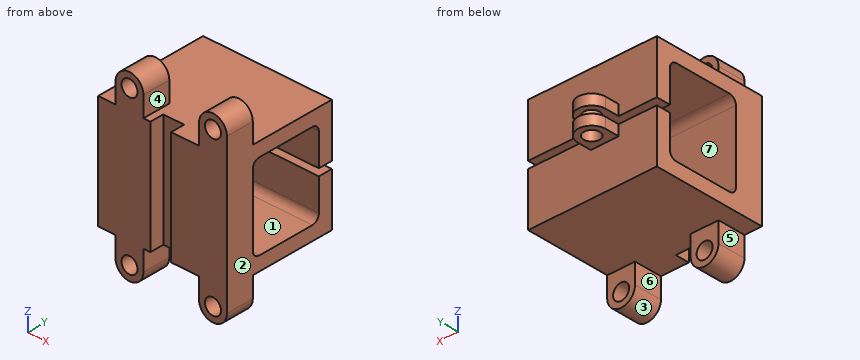
```python
from build123d import *

# Parameters (mm, degrees)
SKETCH_1_W           = 8
SKETCH_1_H           = 5
SKETCH_1_R           = 1.15
EXTRUDE_1_DEPTH      = 4
SKETCH_2_W           = 10.5
SKETCH_2_H           = 8
SKETCH_2_R           = 1.15
EXTRUDE_2_DEPTH      = 7
EXTRUDE_4_DEPTH      = 15
SKETCH_6_R           = 1.15
EXTRUDE_5_DEPTH      = 1.5
EXTRUDE_START        = 2.5
SKETCH_6_2_R         = 1.15
EXTRUDE_6_DEPTH      = 1.5
CUT_EXTRUDE_2_DEPTH  = 3
FILLET_2_R           = 1
SKETCH_9_OUTSIDE_W   = 25.014
SKETCH_9_OUTSIDE_H   = 34.214
SKETCH_9_OUTSIDE_W_2 = 15
SKETCH_9_OUTSIDE_H_2 = 16.2
CUT_EXTRUDE_3_DEPTH  = 36.814522194
SKETCH_12_W          = 16.2
SKETCH_12_H          = 8
CUT_EXTRUDE_5_DEPTH  = 31.608495553
SKETCH_10_W          = 3
SKETCH_10_H          = 2
CUT_EXTRUDE_4_DEPTH  = 31.608495553
SKETCH_11_R          = 1.15
EXTRUDE_7_DEPTH      = 4
EXTRUDE_15_DEPTH     = 3.5


with BuildPart() as part:
    # 草图1 → 凸台-拉伸1 (new body)
    with BuildSketch(Plane(origin=(0, 0, 0), x_dir=(0, 0, -1), z_dir=(1, 0, 0))):
        with Locations((4, 2.5)):
            Rectangle(SKETCH_1_W, SKETCH_1_H)
        with Locations((2, 2.5)):
            Circle(SKETCH_1_R, mode=Mode.SUBTRACT)
        with Locations((6, 2.5)):
            Circle(SKETCH_1_R, mode=Mode.SUBTRACT)
    extrude(amount=EXTRUDE_1_DEPTH)

    # 草图2 → 凸台-拉伸2 (add)
    with BuildSketch(Plane.XZ):
        with Locations((5.25, -4)):
            Rectangle(SKETCH_2_W, SKETCH_2_H)
        with Locations(Location((8, -6, 0), (0, 0, 270))):
            Circle(SKETCH_2_R, mode=Mode.SUBTRACT)
        with Locations(Location((8, -2, 0), (0, 0, 270))):
            Circle(SKETCH_2_R, mode=Mode.SUBTRACT)
    extrude(amount=EXTRUDE_2_DEPTH)

    # 草图5 → 凸台-拉伸4 (add)
    with BuildSketch(Plane.ZY):
        Polygon((14.2, 5), (2, 5), (2, 15.2), (7.6, 15.2), (7.6, 17.2), (0, 17.2), (0, -7), (16.2, -7), (16.2, 17.2), (8.6, 17.2), (8.6, 15.2), (14.2, 15.2), align=None)
    extrude(amount=-EXTRUDE_4_DEPTH)

    # 草图6 → 凸台-拉伸5 (add)
    with BuildSketch(Plane.XY.offset(7.6)):
        with BuildLine():
            Line((2, 19.2), (2, 17.2))
            Line((2, 17.2), (6, 17.2))
            Line((6, 17.2), (6, 19.2))
            ThreePointArc((6, 19.2), (4, 21.2), (2, 19.2))
        make_face()
        with Locations((4, 19.2)):
            Circle(SKETCH_6_R, mode=Mode.SUBTRACT)
    extrude(amount=-EXTRUDE_5_DEPTH)

    # 草图6<2> → 凸台-拉伸6 (add)
    with BuildSketch(Plane.XY.offset(7.6).offset(EXTRUDE_START)):
        with BuildLine():
            Line((2, 19.2), (2, 17.2))
            Line((2, 17.2), (6, 17.2))
            Line((6, 17.2), (6, 19.2))
            ThreePointArc((6, 19.2), (4, 21.2), (2, 19.2))
        make_face()
        with Locations((4, 19.2)):
            Circle(SKETCH_6_2_R, mode=Mode.SUBTRACT)
    extrude(amount=-EXTRUDE_6_DEPTH)

    # 草图8 → 切除-拉伸2 (cut)
    with BuildSketch(Plane(origin=(0, 0, -8), x_dir=(-1, 0, 0), z_dir=(0, 0, -1))):
        Polygon((0, -3), (0, -7), (-4, -7), align=None)
    extrude(amount=-CUT_EXTRUDE_2_DEPTH, mode=Mode.SUBTRACT)

    # 圆角2
    fillet_2_edges = [part.edges().sort_by_distance(p)[0] for p in [
        (7.5, 15.2, 2),
        (7.5, 5, 2),
        (7.5, 5, 14.2),
        (7.5, 15.2, 14.2),
    ]]
    fillet(fillet_2_edges, radius=FILLET_2_R)

    # 草图9 outside → 切除-拉伸3 (cut, through all)
    with BuildSketch(Plane.XZ.offset(7)):
        with Locations((7.5, 4.1)):
            Rectangle(SKETCH_9_OUTSIDE_W, SKETCH_9_OUTSIDE_H)
        with Locations((7.5, 8.1)):
            Rectangle(SKETCH_9_OUTSIDE_W_2, SKETCH_9_OUTSIDE_H_2, mode=Mode.SUBTRACT)
    extrude(amount=-CUT_EXTRUDE_3_DEPTH, mode=Mode.SUBTRACT)

    # 草图12 → 切除-拉伸5 (cut, through all)
    with BuildSketch(Plane(origin=(15, 0, 0), x_dir=(0, 0, -1), z_dir=(1, 0, 0))):
        with Locations((-8.1, -3)):
            Rectangle(SKETCH_12_W, SKETCH_12_H)
    extrude(amount=-CUT_EXTRUDE_5_DEPTH, mode=Mode.SUBTRACT)

    # 草图10 → 切除-拉伸4 (cut, through all)
    with BuildSketch(Plane(origin=(0, 0, 0), x_dir=(-1, 0, 0), z_dir=(0, 0, -1))):
        with Locations((-5.5, 2)):
            Rectangle(SKETCH_10_W, SKETCH_10_H)
    extrude(amount=-CUT_EXTRUDE_4_DEPTH, mode=Mode.SUBTRACT)

    # 草图11 → 凸台-拉伸7 (add)
    # profile 1 of 3: a face of its own
    with BuildSketch(Plane.XZ.offset(-1)):
        with BuildLine():
            Line((0, 16.2), (3, 16.2))
            Line((3, 16.2), (3, 19.1))
            ThreePointArc((3, 19.1), (1, 21.1), (-1, 19.1))
            Line((-1, 19.1), (-1, -2.9))
            ThreePointArc((-1, -2.9), (1, -4.9), (3, -2.9))
            Line((3, -2.9), (3, 0))
            Line((3, 0), (0, 0))
            Line((0, 0), (0, 16.2))
        make_face()
        with Locations(Location((1, 19.1, 0), (0, 0, 270))):
            Circle(SKETCH_11_R, mode=Mode.SUBTRACT)
        with Locations(Location((1, -2.9, 0), (0, 0, 90))):
            Circle(SKETCH_11_R, mode=Mode.SUBTRACT)
    # profile 2 of 3: a face of its own
    with BuildSketch(Plane.XZ.offset(-1)):
        with BuildLine():
            Line((11, 19.1), (11, 16.2))
            Line((11, 16.2), (15, 16.2))
            Line((15, 16.2), (15, 19.1))
            ThreePointArc((15, 19.1), (13, 21.1), (11, 19.1))
        make_face()
        with Locations(Location((13, 19.1, 0), (0, 0, 270))):
            Circle(SKETCH_11_R, mode=Mode.SUBTRACT)
    # profile 3 of 3: a face of its own
    with BuildSketch(Plane.XZ.offset(-1)):
        with BuildLine():
            Line((11, -2.9), (11, 0))
            Line((11, 0), (15, 0))
            Line((15, 0), (15, -2.9))
            ThreePointArc((15, -2.9), (13, -4.9), (11, -2.9))
        make_face()
        with Locations(Location((13, -2.9, 0), (0, 0, 270))):
            Circle(SKETCH_11_R, mode=Mode.SUBTRACT)
    extrude(amount=-EXTRUDE_7_DEPTH)

    # 草图22 → 凸台-拉伸15 (add)
    with BuildSketch(Plane.ZY):
        with BuildLine():
            Line((16.2, 5), (16.2, 17.2))
            Line((16.2, 17.2), (8.6, 17.2))
            Line((8.6, 17.2), (8.6, 15.2))
            Line((8.6, 15.2), (13.2, 15.2))
            ThreePointArc((13.2, 15.2), (13.907106781, 14.907106781), (14.2, 14.2))
            Line((14.2, 14.2), (14.2, 6))
            ThreePointArc((14.2, 6), (13.907106781, 5.292893219), (13.2, 5))
            Line((13.2, 5), (3, 5))
            ThreePointArc((3, 5), (2.292893219, 5.292893219), (2, 6))
            Line((2, 6), (2, 14.2))
            ThreePointArc((2, 14.2), (2.292893219, 14.907106781), (3, 15.2))
            Line((3, 15.2), (7.6, 15.2))
            Line((7.6, 15.2), (7.6, 17.2))
            Line((7.6, 17.2), (0, 17.2))
            Line((0, 17.2), (0, 5))
            Line((0, 5), (0, 1))
            Line((0, 1), (16.2, 1))
            Line((16.2, 1), (16.2, 5))
        make_face()
    extrude(amount=EXTRUDE_15_DEPTH)


solid = part.part
```
Source: CAD feature listing. Evaluate the final solid. Frame: model axes, mm. Face numbers are marked on the shaded views. A direction names the side the tool comes from. Coordinates: 2 decimals unless noted, no trailing zeros. Write each loop counter-clockwise with the first axis right and the second up, starting at its lowest first coordinate (ties: lowest second). Pieces come first, ordered by that corner, then holes. Notation, with made-up numbers: (78, 49) -> (83, 49) arc R26 ccw to (83, 80) -> close; hole circle Ø8 at (9, 43). An arc over 180 degrees is marked (long way). Return JSON: item names as keys, results as strings. Group by question number.
1) Section query C-C, the plane x = 9. Return loops of the section in (y, z).
2) Section query A-A, the plane x = 13. Return loops of the section in (y, z).
3) Section query D-D, the plane x = 3.5. Return loops of the section in (y, z), plus the area to 3 significant figures.
4) Ray query, line 1 along X through (y, z) = (2.4, 19.1); line 2 along X through (y, z) = (3.75, -0.25); line 3 along Y through (x, z) = (10, 12.25). Return the intervals inside material, ascending.
5) Mould query, pull axis X, two halves, no side actions, for the marked faces 1, 2 and 3. Classes: +X half, -X half, draft (parallel to the pull), parting line (faces both ways), or undercut.
6) Contact query for flat-ended pins moving along their axis: P1, Ø1, axis at x = 8.5, y = 9.5, coming from the +Z side; P2, Ø1.4, axis at x = 1, z = -2.9, coming from the +Y side; P3, Ø1.2, axis at y = 18, z = 9, coming from the +X side; P4, Ø6, axis at x = -1.5, y = 14.5, coming from the -Z side. Output: stop coordinate, or through.
7) Section query B-B, the plane z = 1.25. Return loops of the section in (x, y).
8) Set-up query: the marked faces 4, 5, 6 and 7. Return all of +Z, -Z, +X, -X, +Y, -Y with unobstructed straight access to the full face (end or side cutting, diameter ignored); none if empty.
From the geometry:
{
 "1": {"outline": "(1, 0) -> (17.2, 0) -> (17.2, 7.6) -> (15.2, 7.6) -> (15.2, 3) arc R1 cw to (14.2, 2) -> (6, 2) arc R1 cw to (5, 3) -> (5, 13.2) arc R1 cw to (6, 14.2) -> (14.2, 14.2) arc R1 cw to (15.2, 13.2) -> (15.2, 8.6) -> (17.2, 8.6) -> (17.2, 16.2) -> (1, 16.2) -> close"},
 "2": {"outline": "(1, -4.9) -> (5, -4.9) -> (5, -4.05) -> (1, -4.05) -> close; (1, -1.75) -> (5, -1.75) -> (5, 0) -> (17.2, 0) -> (17.2, 7.6) -> (15.2, 7.6) -> (15.2, 3) arc R1 cw to (14.2, 2) -> (6, 2) arc R1 cw to (5, 3) -> (5, 13.2) arc R1 cw to (6, 14.2) -> (14.2, 14.2) arc R1 cw to (15.2, 13.2) -> (15.2, 8.6) -> (17.2, 8.6) -> (17.2, 16.2) -> (5, 16.2) -> (5, 17.95) -> (1, 17.95) -> close; (1, 20.25) -> (5, 20.25) -> (5, 21.1) -> (1, 21.1) -> close"},
 "3": {"outline": "(1, 0) -> (17.2, 0) -> (17.2, 6.1) -> (18.16, 6.1) -> (18.16, 7.6) -> (15.2, 7.6) -> (15.2, 3) arc R1 cw to (14.2, 2) -> (6, 2) arc R1 cw to (5, 3) -> (5, 13.2) arc R1 cw to (6, 14.2) -> (14.2, 14.2) arc R1 cw to (15.2, 13.2) -> (15.2, 8.6) -> (18.16, 8.6) -> (18.16, 10.1) -> (17.2, 10.1) -> (17.2, 16.2) -> (1, 16.2) -> close; (20.24, 6.1) -> (21.14, 6.1) -> (21.14, 7.6) -> (20.24, 7.6) -> close; (20.24, 8.6) -> (21.14, 8.6) -> (21.14, 10.1) -> (20.24, 10.1) -> close", "area": "142 mm²"},
 "4": {"line 1": "-1 to -0.15, 2.15 to 3, 11 to 11.85, 14.15 to 15", "line 2": "-1 to 3, 11 to 15", "line 3": "1 to 5, 15.2 to 17.2"},
 "5": {"face 1": "draft", "face 2": "+X half", "face 3": "undercut"},
 "6": {"P1": "z = 16.2", "P2": "through", "P3": "x = 6", "P4": "z = 0"},
 "7": {"outline": "(-3.5, 1) -> (4, 1) -> (4, 3) -> (7, 3) -> (7, 1) -> (15, 1) -> (15, 17.2) -> (-3.5, 17.2) -> close"},
 "8": {"face 4": "+Z, +Y, -Y", "face 5": "-Z, -X, +Y, -Y", "face 6": "-Z, +Y, -Y", "face 7": "+X, -X"}
}
